```python
from build123d import *

# Parameters (mm, degrees)
F1_DEPTH = 25.4
F2_R     = 6.35
F3_DEPTH = 76.2


with BuildPart() as f1:
    # F0 (on Front) → F1 (new body)
    with BuildSketch(Plane.XZ):
        with BuildLine():
            Line((-12.7, -38.1), (-346.285668, -371.685668))
            ThreePointArc((-346.285668, -371.685668), (-336.867918, -380.242036), (-327.238821, -388.559846))
            ThreePointArc((-327.238821, -388.559846), (468.314664, 196.83845), (-506.569235, 38.1))
            Line((-506.569235, 38.1), (-12.7, 38.1))
            Line((-12.7, 38.1), (481.093702, 38.1))
            ThreePointArc((481.093702, 38.1), (482.6, 0), (481.093702, -38.1))
            Line((481.093702, -38.1), (-12.7, -38.1))
        make_face()
        with BuildLine():
            Line((-309.209041, -370.530065), (-12.7, -74.021024))
            Line((-12.7, -74.021024), (-12.7, -482.432866))
            ThreePointArc((-12.7, -482.432866), (-170.402221, -451.515053), (-309.209041, -370.530065))
        make_face(mode=Mode.SUBTRACT)
        with BuildLine():
            ThreePointArc((478.404128, -63.5), (322.756879, -358.790687), (12.7, -482.432866))
            Line((12.7, -482.432866), (12.7, -63.5))
            Line((12.7, -63.5), (478.404128, -63.5))
        make_face(mode=Mode.SUBTRACT)
        with BuildLine():
            ThreePointArc((-478.404128, 63.5), (-322.756879, 358.790687), (-12.7, 482.432866))
            Line((-12.7, 482.432866), (-12.7, 63.5))
            Line((-12.7, 63.5), (-478.404128, 63.5))
        make_face(mode=Mode.SUBTRACT)
        with BuildLine():
            Line((12.7, 63.5), (12.7, 482.432866))
            ThreePointArc((12.7, 482.432866), (322.756879, 358.790687), (478.404128, 63.5))
            Line((478.404128, 63.5), (12.7, 63.5))
        make_face(mode=Mode.SUBTRACT)
    extrude(amount=F1_DEPTH)

    # F2 (on face) → F3 (join, through all)
    with BuildSketch(Plane.XY.offset(-38.1)):
        with Locations((0, -12.7)):
            Circle(F2_R)
    extrude(amount=F3_DEPTH)


solid = f1.part
```
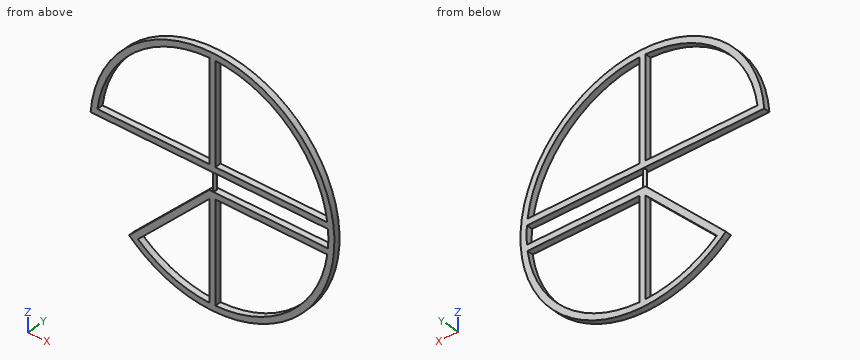
Could you check a few things on this model? Use its own coordinates, in mm. Give positions to 0.01 mm unless a question says otherwise; leave off trailing zeros. Write each loop counter-clockwise with the first axis right and the second up, starting at its lowest first coordinate (ties: lowest second). Pieces come first, ordered by that corner, then holes. Notation, with made-up numbers: (-4, 48.25) -> (4, 48.25) arc R15 cw to (4, 54.25) -> close; hole circle Ø2 at (67.5, -17). An arc over 180 degrees is marked (long way). Write each question's results on one line, items separated by ' | '.
1. I want a section at B-B, the plane y = -12.7. Write out the boundary of the cut face in (x, z), then the cut area to 3 significant figures.
Check sheet entries:
outline: (-506.57, 38.1) -> (-6.35, 38.1) -> (-6.35, -38.1) -> (-12.7, -38.1) -> (-346.29, -371.69) arc R508 ccw to (-327.24, -388.56) arc R508 ccw (long way) to start; hole (-478.4, 63.5) -> (-12.7, 63.5) -> (-12.7, 482.43) arc R482.6 ccw to start; hole (-309.21, -370.53) arc R482.6 ccw to (-12.7, -482.43) -> (-12.7, -74.02) -> close; hole (6.35, -38.1) -> (481.09, -38.1) arc R482.6 ccw to (481.09, 38.1) -> (6.35, 38.1) -> close; hole (12.7, -482.43) arc R482.6 ccw to (478.4, -63.5) -> (12.7, -63.5) -> close; hole (12.7, 63.5) -> (478.4, 63.5) arc R482.6 ccw to (12.7, 482.43) -> close | area: 138,000 mm²
2. I need wall thicknesses on L1, parallel to Z at x = -309.5, y = -2; L2, parallel to X at y = -6.5, z = -197.5; L3, parallel to Z at x = 243, y = -18.75. Which ranges of each line are inside material? Lowest first, please.
Check sheet entries:
L1: z = -402.83 to -334.9, 38.1 to 63.5, 370.29 to 402.83 | L2: x = -172.1 to -136.18, -12.7 to 12.7, 440.34 to 468.04 | L3: z = -446.11 to -416.96, -63.5 to -38.1, 38.1 to 63.5, 416.96 to 446.11
3. I want a section at A-A, the plane z = 0. Write out the boundary of the cut face in (x, y), then the cut area to 3 significant figures.
Check sheet entries:
outline: circle Ø12.7 at (0, -12.7); (482.6, -25.4) -> (508, -25.4) -> (508, 0) -> (482.6, 0) -> close | area: 772 mm²
4. Will these pins go through, and if not, where does the flat tip stop? pin 1 Ø12 at (x, z) = (24, 170) entering from -Y; pin 2 Ø2 at (y, z) = (-9.5, -275) entering from -X; pin 3 Ø8 at (y, z) = (-6, 79) entering from -X; pin 4 Ø7.5 at (x, y) = (351, -16) entering from +Z.
Check sheet entries:
pin 1: passes through | pin 2: stops at x = -250.6 | pin 3: stops at x = -502.43 | pin 4: stops at z = 370.78
5. I want a section at C-C, the plane x = 104.5. Write out the boundary of the cut face in (y, z), then the cut area to 3 significant figures.
Check sheet entries:
outline: (-25.4, -497.14) -> (0, -497.14) -> (0, -471.15) -> (-25.4, -471.15) -> close; (-25.4, -63.5) -> (0, -63.5) -> (0, -38.1) -> (-25.4, -38.1) -> close; (-25.4, 38.1) -> (0, 38.1) -> (0, 63.5) -> (-25.4, 63.5) -> close; (-25.4, 471.15) -> (0, 471.15) -> (0, 497.14) -> (-25.4, 497.14) -> close | area: 2,610 mm²
6. I want a section at D-D, the plane z = 345. Write out the boundary of the cut face in (x, y), then the cut area to 3 significant figures.
Check sheet entries:
outline: (-372.88, -25.4) -> (-337.46, -25.4) -> (-337.46, 0) -> (-372.88, 0) -> close; (-12.7, -25.4) -> (12.7, -25.4) -> (12.7, 0) -> (-12.7, 0) -> close; (337.46, -25.4) -> (372.88, -25.4) -> (372.88, 0) -> (337.46, 0) -> close | area: 2,440 mm²
